The figure shows three views and two pictorial views of one solid part (mm, origin at its lowest corner). Answer the questions. A direction names the side the tool comes from. Give positions to 0.01 mm unless a question says otherwise; leave off trailing zeros. Write each loop counter-clockwise with the first axis right and the second up, starting at its lowest first coordinate (ties: lowest second). Pieces come first, ordered by that corner, then holes. Notation, with made-up numbers: (-33, -4) -> (16, -4) arc R28 ccw to (16, 19) -> close; hole circle Ø5 at (53, 82.25). An arc over 180 degrees is marked (long way). Use a Markdown table: item, result.
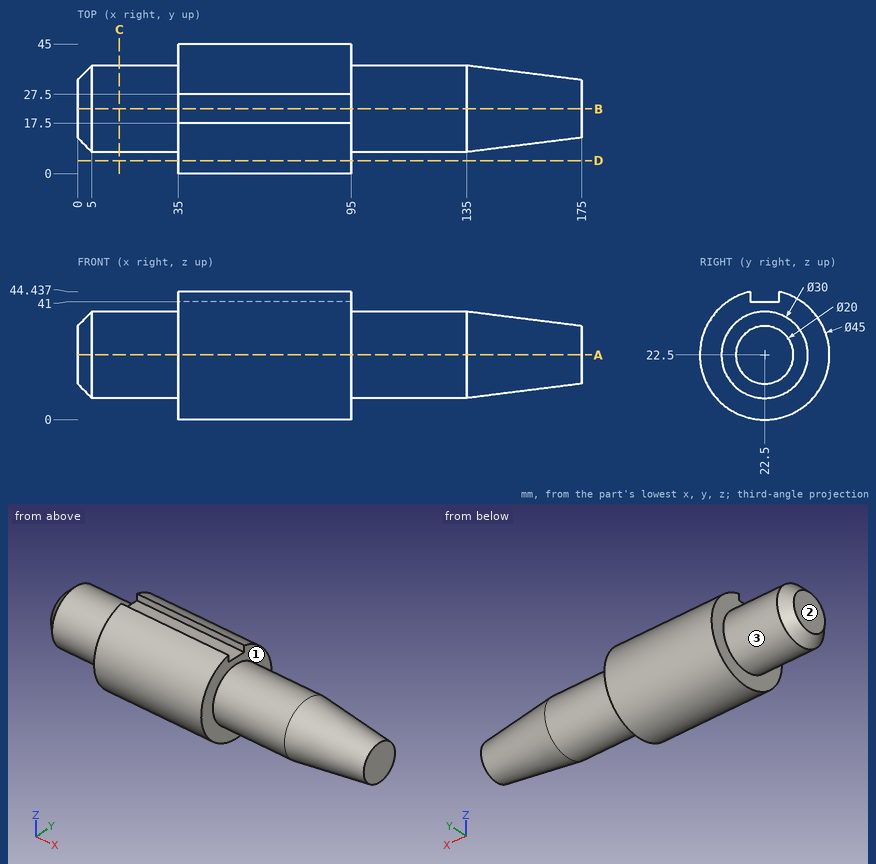
Item 1: A tool of negligible diameter and unlimited length cuts with its end or side. For the marked faces 1, 2 and 3, from which of +Z, -Z, +X, -X, +Y, -Y can it reach the whole face along a straight path? Write none if from no direction.
Return value:
| item | result |
|---|---|
| face 1 | +X |
| face 2 | +Z, -Z, -X, +Y, -Y |
| face 3 | -X |
Item 2: A cutting plane is placed at B-B (y = 22.5). Give the vertices of the cut face in (x, z), then the cut area to 4 significant figures.
Return value:
| item | result |
|---|---|
| outline | (0, 12.5) -> (5, 7.5) -> (35, 7.5) -> (35, 0) -> (95, 0) -> (95, 7.5) -> (135, 7.5) -> (175, 12.5) -> (175, 32.5) -> (135, 37.5) -> (95, 37.5) -> (95, 41) -> (35, 41) -> (35, 37.5) -> (5, 37.5) -> (0, 32.5) -> close |
| area | 5,685 mm^2 |
Item 3: A cutting plane is placed at D-D (y = 4.5). Give the vertices of the cut face in (x, z).
Return value:
| item | result |
|---|---|
| outline | (35, 9) -> (95, 9) -> (95, 36) -> (35, 36) -> close |
Item 4: Straight lines are drawn through the part: line 1 along X through (y, z) = (38.5, 23); line 2 along Y through (x, z) = (92.5, 22) (1 decimal); line 3 along Z through (x, y) = (48.5, 19). For each, find the intervals that lie inside material, in ascending order. Write a range as [from, to].
Return value:
| item | result |
|---|---|
| line 1 | [35, 95] |
| line 2 | [0, 45] |
| line 3 | [0.27, 41] |
Item 5: Each of these flat-tipped pins is pushed along its axis until it touches: P1, Ø12, axis at x = 114, y = 17, coming from the -Z side; P2, Ø8, axis at x = 89, z = 16, coming from the -Y side; P3, Ø2.5, axis at x = 67, z = 42, coming from the -Y side; P4, Ø4, axis at x = 146.5, y = 6, coming from the +Z side. Where does it stop, or does it pass through?
Return value:
| item | result |
|---|---|
| P1 | z = 7.5 |
| P2 | y = 0.14 |
| P3 | y = 9.34 |
| P4 | through |
Item 6: A cutting plane is placed at C-C (x = 14.5). Give the vertices of the cut face in (y, z), then the cut area to 3 significant figures.
Return value:
| item | result |
|---|---|
| outline | circle Ø30 at (22.5, 22.5) |
| area | 707 mm^2 |
Item 7: A cutting plane is placed at A-A (z = 22.5). Give the vertices of the cut face in (x, y).
Return value:
| item | result |
|---|---|
| outline | (0, 12.5) -> (5, 7.5) -> (35, 7.5) -> (35, 0) -> (95, 0) -> (95, 7.5) -> (135, 7.5) -> (175, 12.5) -> (175, 32.5) -> (135, 37.5) -> (95, 37.5) -> (95, 45) -> (35, 45) -> (35, 37.5) -> (5, 37.5) -> (0, 32.5) -> close |
